Autodesk Fusion 360 part; units mm, degrees
sketch "Sketch1" plane through (0, 0, 0) normal (1, 0, 0) x (0, 1, 0)
  line L0 (-20, 20) -> (20, 20) construction
  line L1 (20, 20) -> (20, -20)
  line L2 (20, -20) -> (-20, -20) construction
  line L3 (-20, -20) -> (-20, 20)
  line L4 (0, 0) -> (0, 20) construction
  line L5 (0, 0) -> (20, 0) construction
  line L6 (0, 0) -> (0, -1.6) construction
  line L7 (0, 0) -> (0, -8.6) construction
  circle A0 centre (0, -8.6) radius 6
  circle A1 centre (0, -1.6) radius 18.4 construction
  circle A2 centre (0, -1.6) radius 15.5 construction
  line L8 (0, -1.6) -> (15.5, -1.6) construction
  circle A3 centre (15.5, -1.6) radius 1.5
  circle A4 centre (7.75, 11.8234) radius 1.5
  circle A5 centre (-7.75, 11.8234) radius 1.5
  circle A6 centre (-15.5, -1.6) radius 1.5
  circle A7 centre (-7.75, -15.0234) radius 1.5
  circle A8 centre (7.75, -15.0234) radius 1.5
  line L9 (-10, 20) -> (-10, 24.8) construction
  line L10 (-10, 24.8) -> (10, 24.8)
  line L11 (10, 24.8) -> (10, 20) construction
  line L12 (-10, -20) -> (-10, -24.8) construction
  line L13 (-10, -24.8) -> (10, -24.8)
  line L14 (10, -24.8) -> (10, -20) construction
  line L15 (-11.0607, -21.0607) -> (-10, -20) construction
  line L16 (11.0607, -21.0607) -> (10, -20) construction
  line L17 (-11.0607, 21.0607) -> (-10, 20) construction
  line L18 (11.0607, 21.0607) -> (10, 20) construction
  arc A9 (-12.1213, 20) -> (-10, 22.1213) centre (-11.0607, 21.0607) ccw
  arc A10 (-10, 22.1213) -> (-12.1213, 20) centre (-11.0607, 21.0607) ccw construction
  arc A11 (10, 22.1213) -> (12.1213, 20) centre (11.0607, 21.0607) ccw
  arc A12 (12.1213, 20) -> (10, 22.1213) centre (11.0607, 21.0607) ccw construction
  arc A13 (12.1213, -20) -> (10, -22.1213) centre (11.0607, -21.0607) ccw
  arc A14 (10, -22.1213) -> (12.1213, -20) centre (11.0607, -21.0607) ccw construction
  arc A15 (-10, -22.1213) -> (-12.1213, -20) centre (-11.0607, -21.0607) ccw
  arc A16 (-12.1213, -20) -> (-10, -22.1213) centre (-11.0607, -21.0607) ccw construction
  line L19 (-10, 22.1213) -> (-10, 24.8)
  line L20 (-12.1213, 20) -> (-20, 20)
  line L21 (10, 22.1213) -> (10, 24.8)
  line L22 (12.1213, 20) -> (20, 20)
  line L23 (10, -22.1213) -> (10, -24.8)
  line L24 (12.1213, -20) -> (20, -20)
  line L25 (-10, -22.1213) -> (-10, -24.8)
  line L26 (-12.1213, -20) -> (-20, -20)
  dimension "d61" = 40
  dimension "d62" = 40
  dimension "d63" = 1.6
  dimension "d65" = 12
  dimension "d66" = 36.8
  dimension "d67" = 31
  dimension "d68" = 3
  dimension "d70" = 360
  dimension "d71" = 4.8
  dimension "d72" = 20
  dimension "d73" = 10
  dimension "d74" = 4.8
  dimension "d75" = 20
  dimension "d76" = 10
  dimension "d77" = 3
  dimension "d78" = 1.5
  dimension "d79" = 45
  dimension "d80" = 3
  dimension "d81" = 1.5
  dimension "d83" = 45
  dimension "d84" = 3
  dimension "d85" = 3
  dimension "d86" = 1.5
  dimension "d87" = 45
  dimension "d88" = 1.5
  dimension "d89" = 45
  dimension "d90" = 7
extrude "Extrude1" add sketch "Sketch1" along normal blind 4.8
Design review of the part built by this model. Coordinates are the model's own, in mm. A direction names the side the tool comes from. Round coordinates to 2 decimals unless told otherwise and drop trailing zeros. Write each loop counter-clockwise with the first axis right and the second up, starting at its lowest first coordinate (ties: lowest second). Pieces come first, ordered by that corner, then holes. Notation, with made-up numbers: (74.5, 59) - (94.5, 59) arc R27 cw to (94.5, 81) - close; hole circle Ø4 at (26.5, 38). An arc over 180 degrees is marked (long way). Return JSON: item names as keys, results as strings. Group by question number.
Item 1: Insertion check: P1, Ø0.8, axis at x = 1.5, z = 24, coming from the +Y side; P2, Ø2, axis at x = 2, z = -23, coming from the -Y side; P3, Ø1.4, axis at x = 2, y = 17, coming from the +Z side. Each pin has a flat end and moves straight along its axis. Give the tip position at first contact, or say it passes through.
Item 2: We need section C-C on z = -8.6. Write out the cut boundary in (x, y).
Item 3: We need section B-B on y = -15.5. Write out the cut boundary in (x, z).
Item 4: We need section A-A on z = -1.6. Write out the cut boundary in (x, y), and give its area (3 significant figures).
Item 5: We need section D-D on x = 1.5. Write out the cut boundary in (y, z).
Item 6: Machinability: for faces 5 (the face through (2, -10, -20)), 6 (the face through (2, 10, 23)), 7 (the face through (2, -10, -23)), 8 (the face through (2, -10, 23)), 9 (the face through (2, 16, -20)), which of the approach directions +Z, -Z, +X, -X, +Y, -Y give a long, thin tool a straight path to every point of the face, cutting with its end or side? Answer none if there is none.
Item 7: For probe 1 along Z at (x, y) = (1.95, 7.75); probe 2 along Z at (x, y) = (1.65, -8.5); probe 3 along Z at (x, y) = (2.6, 15.5), list the stretches that pass through material, from the lowest coordinate up. Write a range as [from, to].
Item 8: The part is to be moulded in two halves that separate along Z. For faces 1 (the face through (2, 10, -20)), 2 (the face through (2.37, -17, -1.67)), 3 (the face through (0, 0, 0)), 4 (the face through (2, -16, -20)), say which applies: pulls with the +Z half, pulls with the -Z half, needs draft (parallel to the pull), parting line crosses it, or undercut.
Model answer:
{
 "1": {"P1": "stops at y = 10", "P2": "stops at y = -10", "P3": "stops at z = 20"},
 "2": {"outline": "(0, -20) - (4.8, -20) - (4.8, -6) - (0, -6) - close; (0, 6) - (4.8, 6) - (4.8, 20) - (0, 20) - close"},
 "3": {"outline": "(0, -20) - (4.8, -20) - (4.8, -3.1) - (0, -3.1) - close; (0, -0.1) - (4.8, -0.1) - (4.8, 20) - (0, 20) - close"},
 "4": {"outline": "(0, -20) - (4.8, -20) - (4.8, -17) - (0, -17) - close; (0, -14) - (4.8, -14) - (4.8, 14) - (0, 14) - close; (0, 17) - (4.8, 17) - (4.8, 20) - (0, 20) - close", "area": "163 mm²"},
 "5": {"outline": "(-20, -20) - (-12.12, -20) arc R1.5 cw to (-10, -22.12) - (-10, -24.8) - (10, -24.8) - (10, -22.12) arc R1.5 cw to (12.12, -20) - (20, -20) - (20, 20) - (12.12, 20) arc R1.5 cw to (10, 22.12) - (10, 24.8) - (-10, 24.8) - (-10, 22.12) arc R1.5 cw to (-12.12, 20) - (-20, 20) - close; hole circle Ø3 at (-15.5, -1.6); hole circle Ø3 at (-7.75, -15.02); hole circle Ø3 at (-7.75, 11.82); hole circle Ø12 at (0, -8.6); hole circle Ø3 at (7.75, -15.02); hole circle Ø3 at (7.75, 11.82); hole circle Ø3 at (15.5, -1.6)"},
 "6": {"face 5": "+X, -X", "face 6": "+Z, +X, -X, +Y", "face 7": "-Z, +X, -X, -Y", "face 8": "+Z, +X, -X, -Y", "face 9": "-Z, +X, -X, +Y"},
 "7": {"probe 1": "z = [-24.8, -16.52], [-13.52, 10.32], [13.32, 24.8]", "probe 2": "z = [-24.8, -16.32], [-13.72, 10.52], [13.12, 24.8]", "probe 3": "z = [-20, -3.1], [-0.1, 20]"},
 "8": {"face 1": "undercut", "face 2": "undercut", "face 3": "needs draft", "face 4": "pulls with the -Z half"}
}
